For this review, take the finished solid that the model builds, in its own axes (mm). A direction names the side the tool comes from. Round coordinates to 2 decimals unless told otherwise and drop trailing zeros. Write each loop counter-clockwise with the first axis right and the second up, starting at its lowest first coordinate (ties: lowest second). Pieces come first, ordered by that corner, then holes.
from build123d import *

# Parameters (mm, degrees)
BOSS_EXTRUDE1_DEPTH = 34.29
SKETCH3_W           = 15.24
SKETCH3_H           = 4.445
BOSS_EXTRUDE3_DEPTH = 1.27
SKETCH4_R           = 2.54
CUT_EXTRUDE1_DEPTH  = 7.366092844
SKETCH5_R           = 1.5875
CUT_EXTRUDE2_DEPTH  = 4.175


with BuildPart() as part:
    # Sketch1 → Boss-Extrude1 (new body)
    with BuildSketch(Plane.XY):
        Polygon((3.81, -3.191092844), (-3.81, -3.191092844), (-3.81, -1.667092844), (-6.35, -1.667092844), (-6.35, -0.016092844), (-4.826, -0.016092844), (-4.826, 1.253907156), (-7.62, 1.253907156), (-7.62, -3.191092844), (-15.24, -3.191092844), (-15.24, -6.366092844), (-8.89, -6.366092844), (8.89, -6.366092844), (15.24, -6.366092844), (15.24, -3.191092844), (7.62, -3.191092844), (7.62, 1.253907156), (4.826, 1.253907156), (4.826, -0.016092844), (6.35, -0.016092844), (6.35, -1.667092844), (3.81, -1.667092844), align=None)
    extrude(amount=BOSS_EXTRUDE1_DEPTH)

    # Sketch3 → Boss-Extrude3 (add)
    with BuildSketch(Plane.XY.offset(34.29)):
        with Locations((0, -0.968592844)):
            Rectangle(SKETCH3_W, SKETCH3_H)
    extrude(amount=-BOSS_EXTRUDE3_DEPTH)

    # Sketch4 → Cut-Extrude1 (cut, through all)
    with BuildSketch(Plane(origin=(0, 0, 0), x_dir=(1, 0, 0), z_dir=(0, 1, 0))):
        with Locations((-11.43, -5.08)):
            Circle(SKETCH4_R)
        with Locations((-11.43, -29.21)):
            Circle(SKETCH4_R)
        with Locations((11.43, -29.21)):
            Circle(SKETCH4_R)
        with Locations((11.43, -5.08)):
            Circle(SKETCH4_R)
    extrude(amount=-CUT_EXTRUDE1_DEPTH, mode=Mode.SUBTRACT)

    # Sketch5 → Cut-Extrude2 (cut, through all)
    with BuildSketch(Plane(origin=(0, -3.191092844, 0), x_dir=(1, 0, 0), z_dir=(0, 1, 0))):
        with Locations((0, -3.175)):
            Circle(SKETCH5_R)
    extrude(amount=-CUT_EXTRUDE2_DEPTH, mode=Mode.SUBTRACT)


solid = part.part
(1) We need section B-B, the plane z = 29.21. Give the boundary of the cut face in (x, y), and give its area (3 significant figures).
Geometry check:
outline: (-15.24, -6.37) - (-13.97, -6.37) - (-13.97, -3.19) - (-15.24, -3.19) - close; (-8.89, -6.37) - (8.89, -6.37) - (8.89, -3.19) - (7.62, -3.19) - (7.62, 1.25) - (4.83, 1.25) - (4.83, -0.02) - (6.35, -0.02) - (6.35, -1.67) - (3.81, -1.67) - (3.81, -3.19) - (-3.81, -3.19) - (-3.81, -1.67) - (-6.35, -1.67) - (-6.35, -0.02) - (-4.83, -0.02) - (-4.83, 1.25) - (-7.62, 1.25) - (-7.62, -3.19) - (-8.89, -3.19) - close; (13.97, -6.37) - (15.24, -6.37) - (15.24, -3.19) - (13.97, -3.19) - close
area: 87.4 mm2
(2) For line 1 along X through (y, z) = (-4.05, 29.21); line 2 along Z through (x, y) = (11.43, -5.5); line 3 along X through (y, z) = (-2.25, 6), list the stretches that pass through material, from the lowest coordinate up.
Geometry check:
line 1: x = -15.24 to -13.97, -8.89 to 8.89, 13.97 to 15.24
line 2: z = 0 to 2.54, 7.62 to 26.67, 31.75 to 34.29
line 3: x = -7.62 to -3.81, 3.81 to 7.62
(3) For faces 1 (the face through (7.62, -1, 17)), 2 (the face through (-6.35, -1, 16)), 3 (the face through (-4.826, 1, 16)), list the 3-axis set-ups (+Z, -Z, +X, -X, +Y, -Y) from which the entire face can be reached by the end or side of a thin tool; tool diameter is ignored.
Geometry check:
face 1: +Z, -Z, +X, +Y
face 2: -Z
face 3: -Z, +Y
(4) We need section D-D, the plane y = -0.75. Give the boundary of the cut face in (x, z), and give its area (3 significant figures).
Geometry check:
outline: (-7.62, 0) - (-6.35, 0) - (-6.35, 33.02) - (6.35, 33.02) - (6.35, 0) - (7.62, 0) - (7.62, 34.29) - (-7.62, 34.29) - close
area: 103 mm2
(5) Mouldability with a two-part tool opening along Y and no side actions: class faces 4 (the face through (-6, -0.016, 16)), 5 (the face through (0, -6.366, 17)), 6 (the face through (-3.81, -2, 16)), 7 (the face through (-5, -1.667, 16)) as pulls with the +Y half, pulls with the -Y half, needs draft (parallel to the pull), parting line crosses it, or undercut.
Geometry check:
face 4: undercut
face 5: pulls with the -Y half
face 6: needs draft
face 7: undercut
(6) For pin 1 Ø4 at (x, z) = (-2.5, 9) entering from +Y; pin 2 Ø4.5 at (x, z) = (-11.43, 29.21) entering from -Y; pin 3 Ø1.3 at (y, z) = (-0.5, 14.5) entering from -X; pin 4 Ø8.5 at (x, z) = (11.5, 16) entering from +Y, all flat-tipped, find the tip position at first contact; note any pin that passes through.
Geometry check:
pin 1: stops at y = -1.67
pin 2: passes through
pin 3: stops at x = -7.62
pin 4: stops at y = 1.25
(7) We need section A-A, the plane x = 11.43. Give the boundary of the cut face in (y, z).
Geometry check:
outline: (-6.37, 0) - (-3.19, 0) - (-3.19, 2.54) - (-6.37, 2.54) - close; (-6.37, 7.62) - (-3.19, 7.62) - (-3.19, 26.67) - (-6.37, 26.67) - close; (-6.37, 31.75) - (-3.19, 31.75) - (-3.19, 34.29) - (-6.37, 34.29) - close
(8) We need section C-C, the plane x = 0. Give the boundary of the cut face in (y, z).
Geometry check:
outline: (-6.37, 0) - (-3.19, 0) - (-3.19, 1.59) - (-6.37, 1.59) - close; (-6.37, 4.76) - (-3.19, 4.76) - (-3.19, 33.02) - (1.25, 33.02) - (1.25, 34.29) - (-6.37, 34.29) - close
